```python
from build123d import *

# Parameters (mm, degrees)
SKETCH1_W            = 45
SKETCH1_H            = 50
BOSS_EXTRUDE1_DEPTH  = 16
CUT_EXTRUDE1_DEPTH   = 58.116109812
SKETCH4_W            = 24
SKETCH4_H            = 50
CUT_EXTRUDE2_DEPTH   = 0.72
CUT_EXTRUDE3_DEPTH   = 58.116109812
SKETCH8_R            = 8.05
CUT_EXTRUDE4_DEPTH   = 6
M8_CLEARANCE_HOLE1_D = 8.6
CUT_EXTRUDE5_DEPTH   = 2.5
FILLET1_R            = 1
FILLET2_R            = 1
FILLET4_R            = 0.5
CUT_EXTRUDE7_DEPTH   = 11.5
SKETCH18_R           = 2.75
CUT_EXTRUDE8_DEPTH   = 14.5
SKETCH19_R           = 2.75
CUT_EXTRUDE9_DEPTH   = 10
SKETCH21_W           = 8.99
SKETCH21_H           = 50
BOSS_EXTRUDE2_DEPTH  = 0.6
CHAMFER1_SIZE        = 4
FILLET5_R            = 1
CHAMFER2_SIZE        = 1


with BuildPart() as part:
    # Sketch1 → Boss-Extrude1 (new body)
    with BuildSketch(Plane(origin=(0, 0, 0), x_dir=(1, 0, 0), z_dir=(0, 1, 0))):
        Rectangle(SKETCH1_W, SKETCH1_H)
    extrude(amount=BOSS_EXTRUDE1_DEPTH)

    # Sketch3 → Cut-Extrude1 (cut, through all)
    with BuildSketch(Plane.XY.offset(25)):
        Polygon((-13.5, 16), (-17.5, 12), (22.5, 12), (22.5, 16), align=None)
    extrude(amount=-CUT_EXTRUDE1_DEPTH, mode=Mode.SUBTRACT)

    # Sketch4 → Cut-Extrude2 (cut)
    with BuildSketch(Plane(origin=(0, 12, 0), x_dir=(1, 0, 0), z_dir=(0, 1, 0))):
        with Locations((2.5, 0)):
            Rectangle(SKETCH4_W, SKETCH4_H)
    extrude(amount=-CUT_EXTRUDE2_DEPTH, mode=Mode.SUBTRACT)

    # Sketch5 → Cut-Extrude3 (cut, through all)
    with BuildSketch(Plane.XY.offset(25)):
        Polygon((-22.5, 16), (-13.5, 16), (-13.51, 15.99), (-22.5, 15.99), align=None)
    extrude(amount=-CUT_EXTRUDE3_DEPTH, mode=Mode.SUBTRACT)

    # Sketch8 → Cut-Extrude4 (cut)
    with BuildSketch(Plane(origin=(0, 11.28, 0), x_dir=(1, 0, 0), z_dir=(0, 1, 0))):
        with Locations(Location((-0.5, 0, 0), (0, 0, 180))):
            Circle(SKETCH8_R)
    extrude(amount=-CUT_EXTRUDE4_DEPTH, mode=Mode.SUBTRACT)

    # M8 Clearance Hole1 (through all)
    with Locations(Plane(origin=(0, 5.28, 0), x_dir=(1, 0, 0), z_dir=(0, 1, 0))):
        with Locations((-0.5, 0)):
            Hole(M8_CLEARANCE_HOLE1_D / 2)

    # Sketch12 → Cut-Extrude5 (cut)
    with BuildSketch(Plane(origin=(0, 11.28, 0), x_dir=(1, 0, 0), z_dir=(0, 1, 0))):
        with BuildLine():
            Line((7.5, 16.6), (-2.5, 16.6))
            ThreePointArc((-2.5, 16.6), (-3.207106781, 16.892893219), (-3.5, 17.6))
            Line((-3.5, 17.6), (-3.5, 25))
            Line((-3.5, 25), (8.5, 25))
            Line((8.5, 25), (8.5, 17.6))
            ThreePointArc((8.5, 17.6), (8.207106781, 16.892893219), (7.5, 16.6))
        make_face()
    cut_extrude5 = extrude(amount=-CUT_EXTRUDE5_DEPTH, mode=Mode.SUBTRACT)

    # Fillet1
    fillet1_edges = [part.edges().sort_by_distance(p)[0] for p in [
        (-3.5, 10.03, -25),
        (8.5, 10.03, -25),
    ]]
    fillet(fillet1_edges, radius=FILLET1_R)

    # Mirror2: Cut-Extrude5 across plane
    add(cut_extrude5.mirror(Plane.XY), mode=Mode.SUBTRACT)

    # Fillet2
    fillet2_edges = [part.edges().sort_by_distance(p)[0] for p in [
        (8.207106781, 11.28, 16.892893219),
        (8.5, 11.28, 21.3),
        (-3.5, 11.28, 21.3),
        (-3.207106781, 11.28, 16.892893219),
        (2.5, 11.28, 16.6),
        (-7, 11.28, -25),
        (7.55, 11.28, 0),
        (8.207106781, 11.28, -16.892893219),
        (8.5, 11.28, -20.8),
        (-3.207106781, 11.28, -16.892893219),
        (2.5, 11.28, -16.6),
        (12, 11.28, -25),
        (-3.5, 11.28, -20.8),
        (-3.792893219, 11.28, -24.707106781),
        (8.792893219, 11.28, -24.707106781),
    ]]
    fillet(fillet2_edges, radius=FILLET2_R)

    # Fillet4
    fillet4_edges = [part.edges().sort_by_distance(p)[0] for p in [
        (-17.5, 12, 0),
    ]]
    fillet(fillet4_edges, radius=FILLET4_R)

    # Sketch14 → Cut-Extrude7 (cut)
    with BuildSketch(Plane(origin=(0, 12, 0), x_dir=(1, 0, 0), z_dir=(0, 1, 0))):
        Polygon((19.5, -8), (17.5, -8), (17.5, -3.45), (16.1, -3.45), (16.1, 3.45), (17.5, 3.45), (17.5, 8), (19.5, 8), align=None)
    extrude(amount=-CUT_EXTRUDE7_DEPTH, mode=Mode.SUBTRACT)

    # Sketch18 → Cut-Extrude8 (cut)
    with BuildSketch(Plane(origin=(22.5, 0, 0), x_dir=(0, 0, -1), z_dir=(1, 0, 0))):
        with Locations((0, 6)):
            Circle(SKETCH18_R)
    extrude(amount=-CUT_EXTRUDE8_DEPTH, mode=Mode.SUBTRACT)

    # Sketch19 → Cut-Extrude9 (cut)
    with BuildSketch(Plane(origin=(22.5, 0, 0), x_dir=(0, 0, -1), z_dir=(1, 0, 0))):
        with Locations((-16, 6)):
            Circle(SKETCH19_R)
        with Locations((16, 6)):
            Circle(SKETCH19_R)
    extrude(amount=-CUT_EXTRUDE9_DEPTH, mode=Mode.SUBTRACT)

    # Sketch21 → Boss-Extrude2 (add)
    with BuildSketch(Plane(origin=(0, 15.99, 0), x_dir=(1, 0, 0), z_dir=(0, 1, 0))):
        with Locations((-18.005, 0)):
            Rectangle(SKETCH21_W, SKETCH21_H)
    extrude(amount=BOSS_EXTRUDE2_DEPTH)

    # Chamfer1
    chamfer1_edges = [part.edges().sort_by_distance(p)[0] for p in [
        (-22.5, 8.295, 25),
        (-22.5, 8.295, -25),
    ]]
    chamfer(chamfer1_edges, length=CHAMFER1_SIZE)

    # Fillet5
    fillet5_edges = [part.edges().sort_by_distance(p)[0] for p in [
        (-22.5, 16.59, 0),
    ]]
    fillet(fillet5_edges, radius=FILLET5_R)

    # Chamfer2
    chamfer2_edges = [part.edges().sort_by_distance(p)[0] for p in [
        (18.5, 12, 8),
        (18.5, 12, -8),
    ]]
    chamfer(chamfer2_edges, length=CHAMFER2_SIZE)


solid = part.part
```
Read the model definition and answer for the solid it produces. Units are mm, in the model's axes. A direction names the side the tool comes from. Coordinates: 2 decimals unless noted, no trailing zeros. Write each loop counter-clockwise with the first axis right and the second up, starting at its lowest first coordinate (ties: lowest second). Pieces come first, ordered by that corner, then holes. Notation, with made-up numbers: (-1.75, 34) -> (42.25, 34) arc R19 cw to (42.25, 52) -> close; hole circle Ø5 at (-10.5, 72.25). An arc over 180 degrees is marked (long way). Answer as a JSON object with one key per item and string values.
Q1. The part is cut by section D-D on z = -11.5. Give the vertices of the cut face in (x, y), then the cut area to 3 significant figures.
The answers:
{"outline": "(-22.5, 0) -> (22.5, 0) -> (22.5, 12) -> (14.5, 12) -> (14.5, 11.28) -> (-9.5, 11.28) -> (-9.5, 12) -> (-16.29, 12) arc R0.5 cw to (-16.65, 12.85) -> (-13.51, 15.99) -> (-13.51, 16.59) -> (-21.5, 16.59) arc R1 ccw to (-22.5, 15.59) -> close", "area": "556 mm2"}
Q2. A tool of negligible diameter and unlimited length cuts with its end or side. For faces 5 (the flat face through (8.5, 10, 21)), 6 (the flat face through (12.5, 6, 16)), 7 (the flat face through (8.5, 10, -21)), 8 (the flat face through (17.5, 6, -6)), from which of +Z, -Z, +X, -X, +Y, -Y can it reach the whole face along a straight path? Write none if from no direction.
The answers:
{"face 5": "+Z, +Y", "face 6": "+X", "face 7": "-Z, +Y", "face 8": "+Y"}
Q3. Determine the mould class of faces 1 (the flat face through (14.5, 11.5, 0.3)), 2 (the cylindrical face through (17.57, 4.327, -13.818)), 3 (the flat face through (3, 8.78, 21)), 4 (the cylindrical face through (17.57, 4.327, 18.182)) for opening direction Y: pulls with the +Y half, pulls with the -Y half, needs draft (parallel to the pull), parting line crosses it, or undercut.
The answers:
{"face 1": "needs draft", "face 2": "undercut", "face 3": "pulls with the +Y half", "face 4": "undercut"}
Q4. The part is cut by section A-A on x = -0.5. Give the vertices of the cut face in (y, z), then the cut area to 3 significant figures.
The answers:
{"outline": "(0, -25) -> (8.78, -25) -> (8.78, -16.6) -> (10.28, -16.6) arc R1 ccw to (11.28, -15.6) -> (11.28, -9.05) arc R1 ccw to (10.28, -8.05) -> (5.28, -8.05) -> (5.28, -4.3) -> (0, -4.3) -> close; (0, 4.3) -> (5.28, 4.3) -> (5.28, 8.05) -> (10.28, 8.05) arc R1 ccw to (11.28, 9.05) -> (11.28, 15.6) arc R1 ccw to (10.28, 16.6) -> (8.78, 16.6) -> (8.78, 25) -> (0, 25) -> close", "area": "379 mm2"}
Q5. The part is cut by section B-B on y = 2.5. Give the vertices of the cut face in (x, z).
The answers:
{"outline": "(-22.5, -21) -> (-18.5, -25) -> (22.5, -25) -> (22.5, 25) -> (-18.5, 25) -> (-22.5, 21) -> close; hole circle Ø8.6 at (-0.5, 0); hole (16.1, -3.45) -> (17.5, -3.45) -> (17.5, -8) -> (19.5, -8) -> (19.5, 8) -> (17.5, 8) -> (17.5, 3.45) -> (16.1, 3.45) -> close"}
Q6. Flat-ended cylindrical pins translate along their axes: pin 1 Ø9 at (x, z) = (19, -4.5) entering from +Y; pin 2 Ø10 at (x, z) = (9, -6.5) entering from +Y; pin 3 Ø3.5 at (y, z) = (6, 0) entering from +X. Find the tip coordinate at first contact, or state that the pin passes through.
The answers:
{"pin 1": "stops at y = 12", "pin 2": "stops at y = 11.28", "pin 3": "stops at x = 8"}
Q7. Consider line 1 (X direction, y = 11.5, z = 6.5); line 2 (Y direction, x = 17, z = -16); line 3 (Z direction, x = -0.5, y = 2.75). Determine where each line is inside the solid, lowest interval first. Write a range as [from, to].
The answers:
{"line 1": "x = [-22.5, -9.5], [14.5, 17.5], [19.5, 22.5]", "line 2": "y = [0, 3.25], [8.75, 12]", "line 3": "z = [-25, -4.3], [4.3, 25]"}
